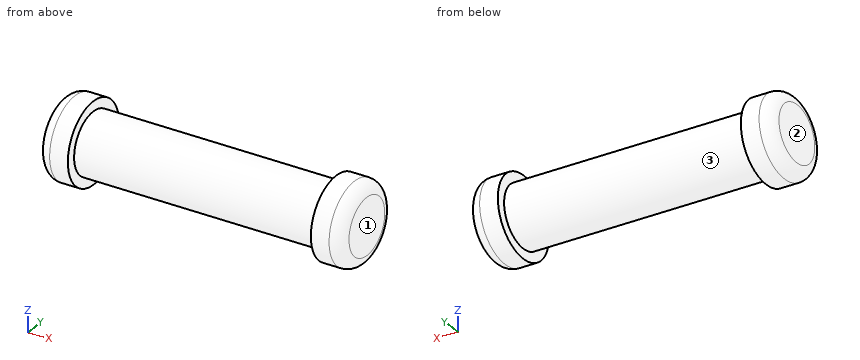
```python
from build123d import *


with BuildPart() as part:
    # Sketch1 → Revolve1 (revolve)
    with BuildSketch(Plane(origin=(0, 0, 0), x_dir=(1, 0, 0), z_dir=(0, 1, 0))):
        with BuildLine():
            Line((-100.780645161, -25.4), (102.419354839, -25.4))
            Line((102.419354839, -25.4), (102.419354839, -33.593548387))
            Line((102.419354839, -33.593548387), (117.659354839, -33.593548387))
            ThreePointArc((117.659354839, -33.593548387), (124.843559736, -30.617753284), (127.819354839, -23.433548387))
            Line((127.819354839, -23.433548387), (127.819354839, 0))
            Line((127.819354839, 0), (-126.180645161, 0))
            Line((-126.180645161, 0), (-126.180645161, -23.433548387))
            ThreePointArc((-126.180645161, -23.433548387), (-123.204850058, -30.617753284), (-116.020645161, -33.593548387))
            Line((-116.020645161, -33.593548387), (-100.780645161, -33.593548387))
            Line((-100.780645161, -33.593548387), (-100.780645161, -25.4))
        make_face()
    revolve(axis=Axis((127.819354839, 0, 0), (-1, 0, 0)))


solid = part.part
```
Here's how the part is built. I have some questions about the finished solid (model axes, mm). Face numbers are marked on the shaded views. Round coordinates to 2 decimals unless told otherwise and drop trailing zeros. Order: outer loops, then holes, each group sorted by start corner. A loop starts at its lowest first (then second) coordinate and runs counter-clockwise, first axis right, second up. Notation, with made-up numbers: M 6.5,76 L 58.5,76 A19 ccw 58.5,98 Z; hole C 0,-6 d10. An arc over 180 degrees is marked long. Use CSV: the item, a comma, the result in double quotes.
1) I need wall thicknesses on line 1 along Z through (x, y) = (-98.5, 1.5); line 2 along X through (y, z) = (-29, -1); line 3 along X through (y, z) = (-24, 10). Which ranges of each line are inside material? Lowest first, please. Write a range as [from, to].
Taken from the geometry:
line 1,"[-25.36, 25.36]"
line 2,"[-124.51, -100.78], [102.42, 126.15]"
line 3,"[-125.85, -100.78], [102.42, 127.49]"
2) I want a section at A-A (y = 0). List the corners of the cut face in (x, z) for me, then the cut area to 3 significant figures.
Taken from the geometry:
outline,"M -126.18,-23.43 A10.16 ccw -116.02,-33.59 L -100.78,-33.59 L -100.78,-25.4 L 102.42,-25.4 L 102.42,-33.59 L 117.66,-33.59 A10.16 ccw 127.82,-23.43 L 127.82,23.43 A10.16 ccw 117.66,33.59 L 102.42,33.59 L 102.42,25.4 L -100.78,25.4 L -100.78,33.59 L -116.02,33.59 A10.16 ccw -126.18,23.43 Z"
area,"13,600 mm^2"
3) I want a section at C-C (x = -76). List the corners of the cut face in (y, z) for me.
Taken from the geometry:
outline,"C 0,0 d50.8"
4) I'm going to push flat-ended pins straight in: P1, Ø6, axis at x = 94.5, y = 15, coming from the -Z side; P2, Ø2, axis at x = -1.5, z = 4, coming from the +Y side; P3, Ø1, axis at x = 93.5, z = -11, coming from the +Y side; P4, Ø1.5, axis at x = -34.5, z = -26.5, coming from the -Y side (3 decimals). Where does each tip first touch, or does it pass through?
Taken from the geometry:
P1,"z = -22.39"
P2,"y = 25.22"
P3,"y = 23.13"
P4,"through"
5) If we mould it in two halves opening along X, with no side actions, what happens to the marked faces 1, 2 and 3? For each: pulls with the +X half, pulls with the -X half, needs draft (parallel to the pull), parting line crosses it, or undercut.
Taken from the geometry:
face 1,"pulls with the +X half"
face 2,"pulls with the -X half"
face 3,"undercut"
